Geometry check sheet. Reference: drawing and pictorial views, mm from the part's lowest x, y, z. Give positions to 0.01 mm unless a question says otherwise; leave off trailing zeros. Write each loop counter-clockwise with the first axis right and the second up, starting at its lowest first coordinate (ties: lowest second). Pieces come first, ordered by that corner, then holes.
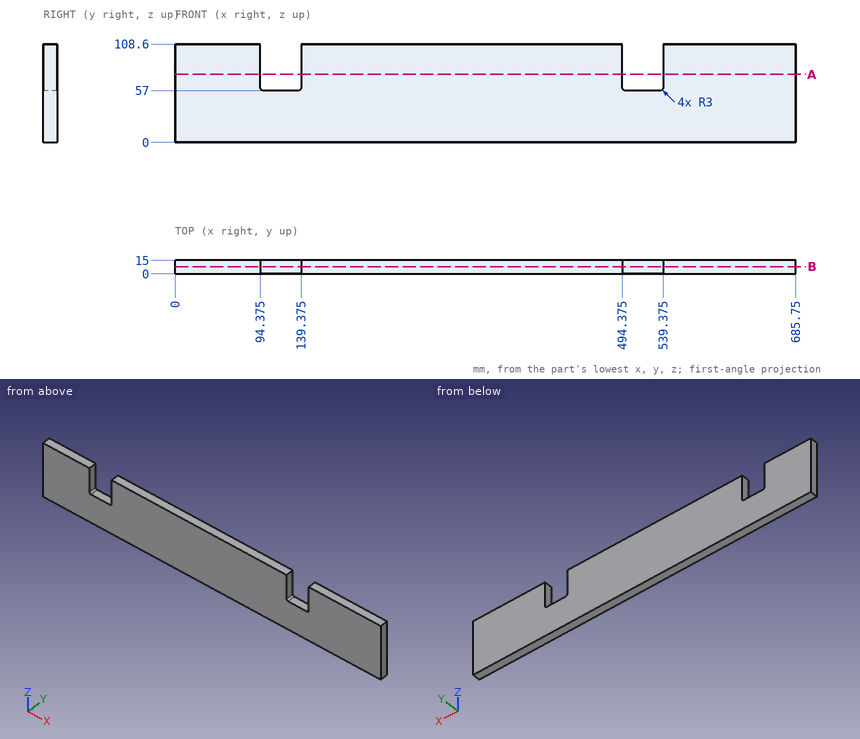
Item 1: Sectioned sample at B-B on y = 8. Record the cut outline in (x, z) (3 decimals), then the cut area to 3 significant figures.
Answer key:
outline: (0, 0) - (685.75, 0) - (685.75, 108.6) - (539.375, 108.6) - (539.375, 60) arc R3 cw to (536.375, 57) - (497.375, 57) arc R3 cw to (494.375, 60) - (494.375, 108.6) - (139.375, 108.6) - (139.375, 60) arc R3 cw to (136.375, 57) - (97.375, 57) arc R3 cw to (94.375, 60) - (94.375, 108.6) - (0, 108.6) - close
area: 69,800 mm2
Item 2: Sectioned sample at A-A on z = 75. Record the cut outline in (x, y) (3 decimals), then the cut area to 3 significant figures.
Answer key:
outline: (0, 0) - (94.375, 0) - (94.375, 15) - (0, 15) - close; (139.375, 0) - (494.375, 0) - (494.375, 15) - (139.375, 15) - close; (539.375, 0) - (685.75, 0) - (685.75, 15) - (539.375, 15) - close
area: 8,940 mm2
Item 3: Scan lines: line 1 along X through (y, z) = (7, 101.5) (3 decimals); line 2 along X through (y, z) = (9, 58); line 3 along Z through (x, y) = (512, 14). Record each from-to range of solid material in increasing order.
Answer key:
line 1: x = 0 to 94.375, 139.375 to 494.375, 539.375 to 685.75
line 2: x = 0 to 95.14, 138.61 to 495.14, 538.61 to 685.75
line 3: z = 0 to 57
